Drawing for the job (mm, zero at the part's lowest x, y, z). Give positions to 0.01 mm unless a question says otherwise; leave off trailing zeros. Order: outer loops, then holes, each group sorted by start corner. A loop starts at its lowest first (then second) coordinate and runs counter-clockwise, first axis right, second up. Notation, with made-up numbers: M 23,3 L 82,3 A4 ccw 82,9 Z; hole C 14,-40 d1. An arc over 180 degrees is marked long. One line per item, written item: value.
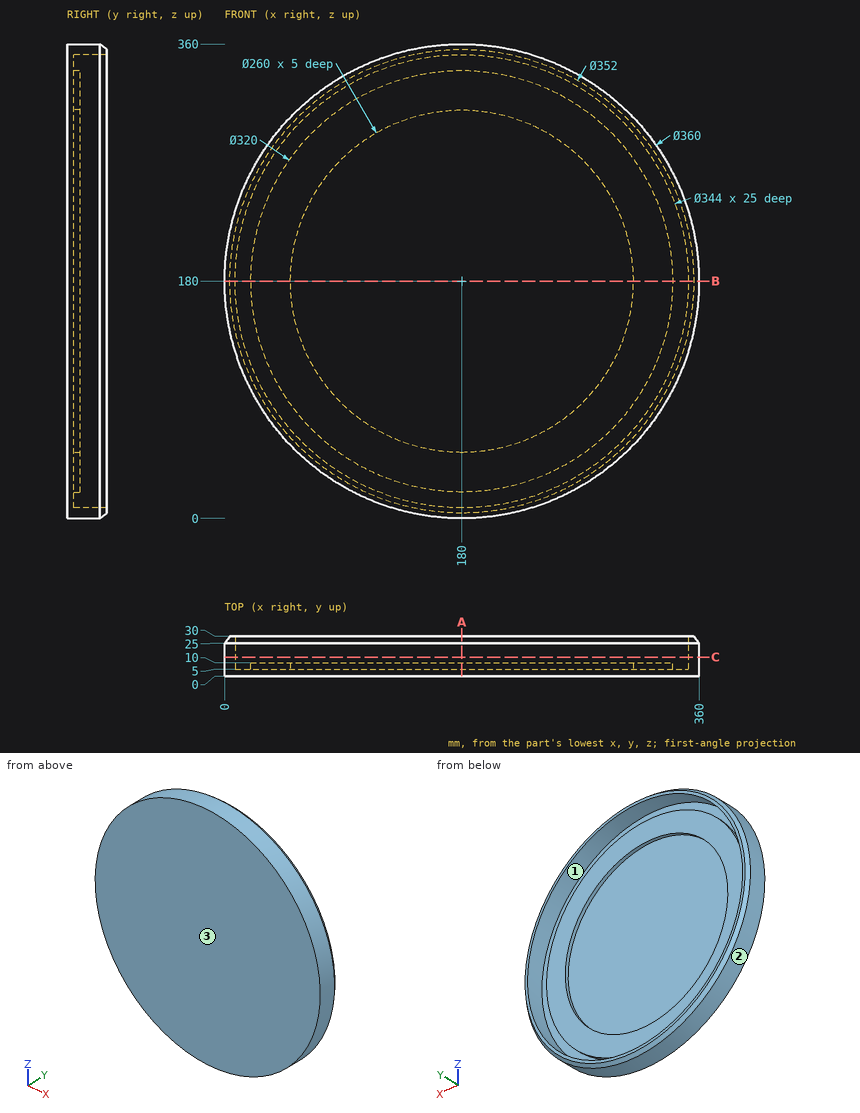
1) Mould opens along Z. For the marked faces 1, 2 and 3 say: released by +Z, released by -Z, zero draft, split by the parting line, or undercut.
Check values:
face 1: undercut
face 2: split by the parting line
face 3: zero draft
2) Saw through at A-A, the plane x = 180. Write the cut outline in (y, z), then the cut area to 3 significant figures.
Check values:
outline: M 0,0 L 25,0 L 30,4 L 30,8 L 5,8 L 5,20 L 10,20 L 10,50 L 5,50 L 5,310 L 10,310 L 10,340 L 5,340 L 5,352 L 30,352 L 30,356 L 25,360 L 0,360 Z
area: 2,480 mm^2
3) Saw through at C-C, the plane y = 14.25. Write the cut outline in (x, z).
Check values:
outline: C 180,180 d360; hole C 180,180 d344
4) Pin check, flat tips, straight feed: pin 1 (4 mm diameter, centred on x = 58, y = 15.5, fed in from +Z); pin 2 (1.5 mm diameter, centred on x = 235.5, y = 13, fed in from +Z); pin 3 (8 mm diameter, centred on x = 172.5, z = 59, fed in from +Y). Stop position of each tip, or through.
Check values:
pin 1: z = 314.16
pin 2: z = 351.47
pin 3: y = 5
5) Saw through at B-B, the plane z = 180. Write the cut outline in (x, y), then the cut area to 3 significant figures.
Check values:
outline: M 0,0 L 360,0 L 360,25 L 356,30 L 352,30 L 352,5 L 340,5 L 340,10 L 310,10 L 310,5 L 50,5 L 50,10 L 20,10 L 20,5 L 8,5 L 8,30 L 4,30 L 0,25 Z
area: 2,480 mm^2
6) Drill centre lines: probe 1 along X at (y, z) = (7.85, 180); probe 2 along Z at (x, y) = (178.5, 12); probe 3 along X at (y, z) = (24, 180). Where is each one in solid material? Low to high. Write a range as from..to.
Check values:
probe 1: 0..8, 20..50, 310..340, 352..360
probe 2: 0.01..8.01, 351.99..359.99
probe 3: 0..8, 352..360
